```python
from build123d import *

# Parameters (mm, degrees)
SKETCH1_W           = 341
SKETCH1_H           = 220
BOSS_EXTRUDE1_DEPTH = 1
SKETCH2_R           = 8.25
CUT_EXTRUDE1_DEPTH  = 203.906998401
SKETCH3_R           = 3
CUT_EXTRUDE2_DEPTH  = 203.906998401


with BuildPart() as part:
    # Sketch1 → Boss-Extrude1 (new body)
    with BuildSketch(Plane.YZ):
        Rectangle(SKETCH1_W, SKETCH1_H)
    extrude(amount=BOSS_EXTRUDE1_DEPTH)

    # Sketch2 → Cut-Extrude1 (cut, through all)
    with BuildSketch(Plane.YZ.offset(1)):
        with Locations(Location((150.50261802, 50, 0), (0, 0, 270))):
            Circle(SKETCH2_R)
        with Locations(Location((150.50261802, 16.67, 0), (0, 0, 270))):
            Circle(SKETCH2_R)
        with Locations(Location((150.50261802, -16.67, 0), (0, 0, 90))):
            Circle(SKETCH2_R)
        with Locations(Location((150.50261802, -50, 0), (0, 0, 90))):
            Circle(SKETCH2_R)
        with Locations(Location((-150.50261802, -50, 0), (0, 0, 270))):
            Circle(SKETCH2_R)
        with Locations(Location((-150.50261802, -16.67, 0), (0, 0, 270))):
            Circle(SKETCH2_R)
        with Locations(Location((-150.50261802, 16.67, 0), (0, 0, 90))):
            Circle(SKETCH2_R)
        with Locations(Location((-150.50261802, 50, 0), (0, 0, 90))):
            Circle(SKETCH2_R)
        with BuildLine():
            Line((-130.50261802, 91.002659242), (-130.502618018, -91.002659141))
            ThreePointArc((-130.502618018, -91.002659141), (-129.477508731, -93.477508839), (-127.002658987, -94.502618015))
            Line((-127.002658987, -94.502618015), (127.002659141, -94.502618018))
            ThreePointArc((127.002659141, -94.502618018), (129.477508787, -93.477508786), (130.50261802, -91.002659141))
            Line((130.50261802, -91.002659141), (130.502618017, 91.002659141))
            ThreePointArc((130.502618017, 91.002659141), (129.477508731, 93.477508839), (127.002658987, 94.502618015))
            Line((127.002658987, 94.502618015), (-127.00265914, 94.502618018))
            ThreePointArc((-127.00265914, 94.502618018), (-129.477508751, 93.477508822), (-130.50261802, 91.002659242))
        make_face()
    extrude(amount=-CUT_EXTRUDE1_DEPTH, mode=Mode.SUBTRACT)

    # Sketch3 → Cut-Extrude2 (cut, through all)
    with BuildSketch(Plane.YZ.offset(1)):
        with Locations(Location((-160.5, 100, 0), (0, 0, 270))):
            Circle(SKETCH3_R)
        with Locations(Location((160.5, 100, 0), (0, 0, 90))):
            Circle(SKETCH3_R)
        with Locations(Location((-160.5, -100, 0), (0, 0, 90))):
            Circle(SKETCH3_R)
        with Locations(Location((160.5, -100, 0), (0, 0, 270))):
            Circle(SKETCH3_R)
    extrude(amount=-CUT_EXTRUDE2_DEPTH, mode=Mode.SUBTRACT)


solid = part.part
```
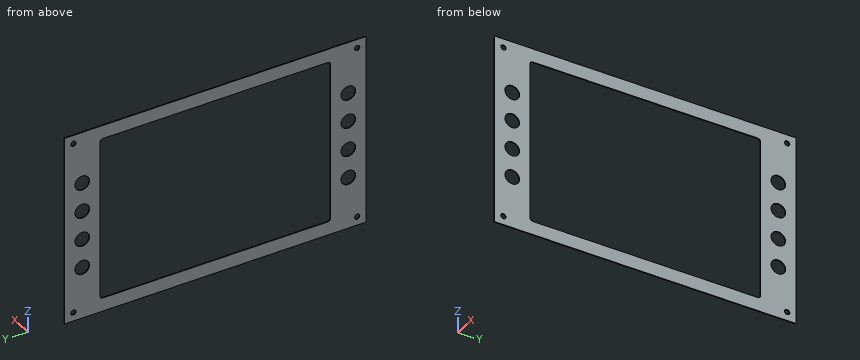
The model under review builds one solid part; all positions refer to its coordinate system, in mm. Round coordinates to 2 decimals unless told otherwise and drop trailing zeros. Order: outer loops, then holes, each group sorted by start corner. A loop starts at its lowest first (then second) coordinate and runs counter-clockwise, first axis right, second up. Notation, with made-up numbers: M 25,66.25 L 56,66.25 A22 cw 56,104.25 Z; hole C 8,-13 d6. An arc over 180 degrees is marked long. Use a Markdown table: item, result.
1) Wall thickness on line 1 along Y through (x, z) = (0.5, -50); line 2 along Z through (x, y) = (0.3, -160.5); line 3 along Y through (x, z) = (0.3, 100): over which ranges is each line inside the solid? List them lowest first. Write a range as [from, to].
Report:
| item | result |
|---|---|
| line 1 | [-170.5, -158.75], [-142.25, -130.5], [130.5, 142.25], [158.75, 170.5] |
| line 2 | [-110, -103], [-97, 97], [103, 110] |
| line 3 | [-170.5, -163.5], [-157.5, 157.5], [163.5, 170.5] |
2) Consider section C-C (z = 65). Write out the cut boundary in (x, y), then the cut area to 3 significant figures.
Report:
| item | result |
|---|---|
| outline | M 0,-170.5 L 1,-170.5 L 1,-130.5 L 0,-130.5 Z; M 0,130.5 L 1,130.5 L 1,170.5 L 0,170.5 Z |
| area | 80.0 mm^2 |
3) Consider section B-B (z = 16.67). Write out the cut boundary in (x, y), then the cut area to 3 significant figures.
Report:
| item | result |
|---|---|
| outline | M 0,-170.5 L 1,-170.5 L 1,-158.75 L 0,-158.75 Z; M 0,-142.25 L 1,-142.25 L 1,-130.5 L 0,-130.5 Z; M 0,130.5 L 1,130.5 L 1,142.25 L 0,142.25 Z; M 0,158.75 L 1,158.75 L 1,170.5 L 0,170.5 Z |
| area | 47.0 mm^2 |
4) Consider section A-A (y = -51.5). Write out the cut boundary in (x, z).
Report:
| item | result |
|---|---|
| outline | M 0,-110 L 1,-110 L 1,-94.5 L 0,-94.5 Z; M 0,94.5 L 1,94.5 L 1,110 L 0,110 Z |
5) Consider section D-D (x = 0.25). Give the number of separate pieces and of enclosed holes in the cut face, then the cut area to 3 significant figures.
Report:
| item | result |
|---|---|
| separate pieces | 1 |
| enclosed holes | 13 |
| area | 23,900 mm^2 |
6) Insertion check: pin 1 (15 mm diameter, centred on y = -150.5, z = -50, fed in from -X). The pin has a flat end and moves straight along its axis. Give the tip position at first contact, or say it passes through.
Report:
| item | result |
|---|---|
| pin 1 | through |
